Geometry check sheet. Reference: the model listing, model coordinates, mm. Face numbers are marked on the shaded views. A direction names the side the tool comes from. Give positions to 0.01 mm unless a question says otherwise; leave off trailing zeros. Order: outer loops, then holes, each group sorted by start corner. A loop starts at its lowest first (then second) coordinate and runs counter-clockwise, first axis right, second up. Notation, with made-up numbers: M 31.25,37 L 52.25,37 A35 cw 52.25,70 Z; hole C 39.25,48 d1. An arc over 180 degrees is marked long. Answer as CSV lines item,"result".
from build123d import *

# Parameters (mm, degrees)
F1_DEPTH      = 10
F3_DEPTH      = 20.001
F3_DEPTH_BACK = 197
F4_R          = 1.5
F5_DEPTH      = 1.5
F4_R_2        = 4.25
F6_DEPTH      = 112.584302492
F4_R_3        = 5.5
F7_DEPTH      = 2
F8_W          = 17
F8_H          = 6
F9_DEPTH      = 10.001
F10_W         = 7
F10_H         = 8
F11_DEPTH     = 4


# Not quite as in the source:
# - an extrude ends at something that could not be found from the text; its depth is read off the source's solid


with BuildPart() as f1:
    # F0 (on Front) → F1 (new body, symmetric)
    with BuildSketch(Plane.XZ):
        with BuildLine():
            Line((30, 51.9615242271), (0, 0))
            Line((0, 0), (130, 0))
            Line((130, 0), (130, 10))
            Line((130, 10), (88.0384757729, 10))
            ThreePointArc((88.0384757729, 10), (82.8620948709, 10.6814834742), (78.0384757729, 12.6794919243))
            Line((78.0384757729, 12.6794919243), (62.2390923627, 21.8012701892))
            ThreePointArc((62.2390923627, 21.8012701892), (61.5402036233, 22.7120797272), (61.6900542571, 23.8503082949))
            Line((61.6900542571, 23.8503082949), (62.1900542571, 24.7163336987))
            Line((62.1900542571, 24.7163336987), (44.8695461814, 34.7163336987))
            Line((44.8695461814, 34.7163336987), (44.3695461814, 33.8503082949))
            ThreePointArc((44.3695461814, 33.8503082949), (43.4587366433, 33.1514195555), (42.3205080757, 33.3012701892))
            Line((42.3205080757, 33.3012701892), (27.5980762114, 41.8012701892))
            ThreePointArc((27.5980762114, 41.8012701892), (26.8991874719, 42.7120797272), (27.0490381057, 43.8503082949))
            Line((27.0490381057, 43.8503082949), (31.2990381057, 51.2115242271))
            Line((31.2990381057, 51.2115242271), (30, 51.9615242271))
        make_face()
        with BuildLine():
            ThreePointArc((23.0490381057, 36.9221050646), (26.0850698991, 39.2517341961), (29.8791651246, 38.7522320835))
            Line((29.8791651246, 38.7522320835), (78.2416697508, 10.8301270189))
            ThreePointArc((78.2416697508, 10.8301270189), (80.5712988822, 5.2059047745), (75.7416697508, 1.5))
            Line((75.7416697508, 1.5), (27.4019237886, 1.5))
            Line((27.4019237886, 1.5), (13.1291651246, 9.7403810568))
            ThreePointArc((13.1291651246, 9.7403810568), (10.7995359932, 12.7764128502), (11.2990381057, 16.5705080757))
            Line((11.2990381057, 16.5705080757), (23.0490381057, 36.9221050646))
        make_face(mode=Mode.SUBTRACT)
        with BuildLine():
            Line((78.2416697508, 10.8301270189), (29.8791651246, 38.7522320835))
            ThreePointArc((29.8791651246, 38.7522320835), (26.0850698991, 39.2517341961), (23.0490381057, 36.9221050646))
            Line((23.0490381057, 36.9221050646), (11.2990381057, 16.5705080757))
            ThreePointArc((11.2990381057, 16.5705080757), (10.7995359932, 12.7764128502), (13.1291651246, 9.7403810568))
            Line((13.1291651246, 9.7403810568), (27.4019237886, 1.5))
            Line((27.4019237886, 1.5), (75.7416697508, 1.5))
            ThreePointArc((75.7416697508, 1.5), (80.5712988822, 5.2059047745), (78.2416697508, 10.8301270189))
        make_face()
    extrude(amount=F1_DEPTH, both=True)

    # F2 (on face) → F3 (cut, two sides)
    with BuildSketch(Plane.XZ.offset(10)) as f3_sk:
        with BuildLine():
            ThreePointArc((29.8791651246, 38.7522320835), (26.0850698991, 39.2517341961), (23.0490381057, 36.9221050646))
            Line((23.0490381057, 36.9221050646), (11.2990381057, 16.5705080757))
            ThreePointArc((11.2990381057, 16.5705080757), (10.7995359932, 12.7764128502), (13.1291651246, 9.7403810568))
            Line((13.1291651246, 9.7403810568), (27.4019237886, 1.5))
            Line((27.4019237886, 1.5), (75.7416697508, 1.5))
            ThreePointArc((75.7416697508, 1.5), (80.5712988822, 5.2059047745), (78.2416697508, 10.8301270189))
            Line((78.2416697508, 10.8301270189), (29.8791651246, 38.7522320835))
        make_face()
    extrude(amount=-F3_DEPTH, mode=Mode.SUBTRACT)
    extrude(f3_sk.sketch, amount=F3_DEPTH_BACK, mode=Mode.SUBTRACT)

    # F4 (on face) → F5 (cut, through all)
    with BuildSketch(Plane(origin=(0, 0, 0), x_dir=(0, -1, 0), z_dir=(-0.8660254038, 0, 0.5))):
        with Locations((-5, 25)):
            Circle(F4_R)
        with Locations((-5, 32)):
            Circle(F4_R)
        with Locations((-5, 39)):
            Circle(F4_R)
        with Locations((5, 39)):
            Circle(F4_R)
        with Locations((5, 32)):
            Circle(F4_R)
        with Locations((5, 25)):
            Circle(F4_R)
    extrude(amount=-F5_DEPTH, mode=Mode.SUBTRACT)

    # F4 (on face) → F6 (cut, through all)
    with BuildSketch(Plane(origin=(0, 0, 0), x_dir=(0, -1, 0), z_dir=(-0.8660254038, 0, 0.5))):
        with Locations((0, 10)):
            Circle(F4_R_2)
    extrude(amount=-F6_DEPTH, mode=Mode.SUBTRACT)

    # F4 (on face) → F7 (cut)
    with BuildSketch(Plane(origin=(0, 0, 0), x_dir=(0, -1, 0), z_dir=(-0.8660254038, 0, 0.5))):
        with Locations((0, 10)):
            Circle(F4_R_3)
        with Locations((0, 10)):
            Circle(F4_R_2, mode=Mode.SUBTRACT)
    extrude(amount=-F7_DEPTH, mode=Mode.SUBTRACT)

    # F8 (on face) → F9 (cut, through all)
    with BuildSketch(Plane.XY.offset(10)):
        with Locations((121.5, 0)):
            Rectangle(F8_W, F8_H)
        with BuildLine():
            ThreePointArc((113, 3), (110, 0), (113, -3))
            Line((113, -3), (113, 3))
        make_face()
        with BuildLine():
            Line((130, -10), (130, -5))
            Line((130, -5), (98, -5))
            ThreePointArc((98, -5), (95.8786796564, -5.8786796564), (95, -8))
            Line((95, -8), (95, -10))
            Line((95, -10), (130, -10))
        make_face()
        with BuildLine():
            Line((98, 5), (130, 5))
            Line((130, 5), (130, 10))
            Line((130, 10), (95, 10))
            Line((95, 10), (95, 8))
            ThreePointArc((95, 8), (95.8786796564, 5.8786796564), (98, 5))
        make_face()
    extrude(amount=-F9_DEPTH, mode=Mode.SUBTRACT)

    # F10 (on face) → F11 (cut, through all)
    with BuildSketch(Plane(origin=(26.25, 0, 45.4663336987), x_dir=(0.8660254038, 0, -0.5), z_dir=(0.5, 0, 0.8660254038))):
        with BuildLine():
            ThreePointArc((28, 4), (24, 0), (28, -4))
            Line((28, -4), (28, 4))
        make_face()
        with Locations((31.5, 0)):
            Rectangle(F10_W, F10_H)
        with BuildLine():
            Line((35, 4), (35, -4))
            ThreePointArc((35, -4), (39, 0), (35, 4))
        make_face()
    extrude(amount=-F11_DEPTH, mode=Mode.SUBTRACT)


solid = f1.part
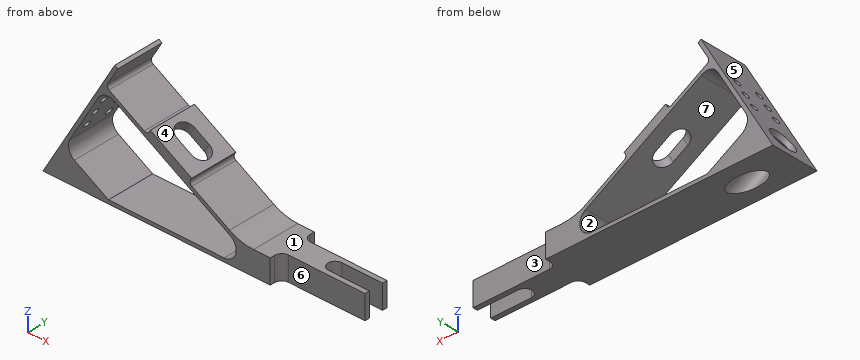
(1) Draft check along X on the marked faces 4, 5, 6 and 7. Enter one of: +X half, -X half, draft (parallel to the pull), parting line (faces both ways), or undercut.
The answers:
face 4,"+X half"
face 5,"-X half"
face 6,"draft"
face 7,"undercut"
(2) Tool access check on the marked faces 1, 2 and 3. Record the directions out of +Z, -Z, +X, -X, +Y, -Y that give a thin tool (end or side, any length) a straight path to the whole face; none if there is none.
The answers:
face 1,"+Z, +X, +Y, -Y"
face 2,"+Y, -Y"
face 3,"+Z, -Z, +X, +Y"
(3) Section check B-B on x = 93. Enter the section's corners in (y, z), then the cut area to 3 significant figures.
The answers:
outline,"M -10,0 L 10,0 L 10,10 L -10,10 Z"
area,"200 mm2"
(4) Material ranges on line 1 (X direction, y = 8, z = 17); line 2 (Y direction, x = 113, z = 3.5); line 3 (X direction, y = 9, z = 32), recorded low to high.
The answers:
line 1,"x = 9.81 to 11.55, 67.56 to 70.56"
line 2,"y = -5 to -3, 3 to 5"
line 3,"x = 18.48 to 20.21, 41.57 to 49.57"
(5) Gauge pin test, flat ends, axial feed: P1, Ø5, axis at y = -5.5, z = 44, coming from the -X side; P2, Ø5, axis at x = 120.5, z = 4.5, coming from the -Y side; P3, Ø2, axis at y = 4, z = 34.5, coming from the +X side. Record the tip position at first contact, or that the pin passes through.
The answers:
P1,"stops at x = 23.96"
P2,"stops at y = -5"
P3,"stops at x = 46.98"
